Read the model definition and answer for the solid it produces. Units are mm, in the model's axes. A direction names the side the tool comes from. Round coordinates to 2 decimals unless told otherwise and drop trailing zeros. Order: outer loops, then holes, each group sorted by start corner. A loop starts at its lowest first (then second) coordinate and runs counter-clockwise, first axis right, second up. Notation, with made-up numbers: (31, 68.5) -> (49, 68.5) arc R18 ccw to (49, 86.5) -> close; hole circle Ø3 at (39.25, 5). An arc over 180 degrees is marked (long way). One line per item, written item: value. Start each with the question number.
1. Section D-D (x = 122) is taken. Give the vertices of the cut face in (y, z).
2. Consider line 1 (Y direction, x = 39, z = 70.5); line 2 (Z direction, x = -78, y = -39.5); line 3 (X direction, y = -22, z = 64.5). Determine where each line is inside the solid, lowest interval first.
3. Flat-ended cylindrical pins translate along their axes: pin 1 Ø1 at (x, z) = (171.5, 4.5) entering from +Y; pin 2 Ø1 at (x, z) = (-25, 78) entering from +Y; pin 3 Ø1.6 at (y, z) = (-37.5, 128.5) entering from +X; pin 4 Ø6 at (x, z) = (63, 39) entering from -Y. Find the tip coordinate at first contact, or state that the pin passes through.
4. Section C-C (y = -61) is taken. Give the vertices of the cut face in (x, z) (3 decimals).
5. For faces 1 (the face through (-24, -56, 130.175)), 2 (the face through (-8, -38, -3.175)), 3 (the face through (-60.93, -57.73, -1.88)), determine the directions among +Z, -Z, +X, -X, +Y, -Y from which every point of the face is accessible in a straight line to the end or side of a thin tool.
6. Section B-B (z = 38.5) is taken. Give the vertices of the cut face in (x, y), then the cut area to 3 significant figures.
7. Section A-A (x = -29.5) is taken. Give the vertices of the cut face in (y, z) (3 decimals), then the cut area to 3 significant figures.
from build123d import *

# Parameters (mm, degrees)
F5_DEPTH  = 127
F6_W      = 54.5970508829
F6_H      = 20.5464081178
F7_DEPTH  = 3.81
F8_W      = 15.3487510979
F8_H      = 7.4063618667
F8_H_2    = 7.1164776087
F9_DEPTH  = 3.175
F10_W     = 10.7039126975
F10_H     = 8.7776441574
F10_H_2   = 9.3331737444
F11_DEPTH = 3.175
F12_W     = 40.7254230231
F12_H     = 18.2523988187
F12_W_2   = 46.4485138655
F13_DEPTH = 3.175
F14_W     = 15.8928539604
F14_H     = 6.1111226678
F14_W_2   = 13.3333727717
F14_H_2   = 5.5555664003
F15_DEPTH = 3.175
F16_W     = 11.666694656
F16_H     = 5.5555701256
F16_W_2   = 12.222263962
F17_DEPTH = 3.175


# Not quite as in the source:
# - the program builds the solid bodies; features that only make, move or delete a surface that nothing else refers to are left out


with BuildPart() as f5:
    # F0 (on Top) → F5 (new body)
    with BuildSketch(Plane.XY):
        with BuildLine():
            Line((94.2318475405, -7.3630477542), (-68.6407278484, -7.3630477542))
            ThreePointArc((-68.6407278484, -7.3630477542), (-68.7653713247, -7.3626377944), (-68.8900094076, -7.3614079328))
            Line((-68.8900094076, -7.3614079328), (-88.84768188, -7.2301225737))
            Line((-88.84768188, -7.2301225737), (-120.7322572041, -7.2301225737))
            Line((-120.7322572041, -7.2301225737), (-151.5727639198, -17.6438004827))
            Line((-151.5727639198, -17.6438004827), (-151.5727639198, -39.0516258776))
            Line((-151.5727639198, -39.0516258776), (-80.8923020959, -47.3129786551))
            Line((-80.8923020959, -47.3129786551), (-46.3170148432, -70.5671533942))
            Line((-46.3170148432, -70.5671533942), (62.6104325056, -70.5671533942))
            Line((62.6104325056, -70.5671533942), (117.5853461027, -47.3129786551))
            Line((117.5853461027, -47.3129786551), (170.3427284956, -47.3129786551))
            Line((170.3427284956, -47.3129786551), (170.3427284956, -19.2245114595))
            Line((170.3427284956, -19.2245114595), (127.9769688845, -7.2301225737))
            Line((127.9769688845, -7.2301225737), (94.2318475405, -7.3630477542))
        make_face()
    extrude(amount=F5_DEPTH)

    # F6 (on face) → F7 (join)
    with BuildSketch(Plane(origin=(0, 0, 0), x_dir=(1, 0, 0), z_dir=(0, 0, -1))):
        Polygon((-45.8669510931, 67.8593867729), (-76.4162167907, 47.3129786551), (0, 47.3129786551), (0, 67.8593867729), align=None)
        with Locations((35.3119070642, 57.586182714)):
            Rectangle(F6_W, F6_H)
    extrude(amount=F7_DEPTH)

    # F8 (on face) → F9 (join)
    with BuildSketch(Plane.YZ.offset(170.3427284956)):
        with Locations((-39.6386031061, 3.7031809334)):
            Rectangle(F8_W, F8_H)
        with Locations((-39.6386031061, 123.4417611957)):
            Rectangle(F8_W, F8_H_2)
    extrude(amount=F9_DEPTH)

    # F10 (on face) → F11 (join)
    with BuildSketch(Plane(origin=(-151.5727639198, 0, 0), x_dir=(0, -1, 0), z_dir=(-1, 0, 0))):
        with Locations((33.6996695289, 122.6111779213)):
            Rectangle(F10_W, F10_H)
        with Locations((33.6996695289, 4.6665868722)):
            Rectangle(F10_W, F10_H_2)
    extrude(amount=F11_DEPTH)

    # F12 (on face) → F13 (join)
    with BuildSketch(Plane.XY.offset(127)):
        with Locations((42.2477209941, -56.4391780645)):
            Rectangle(F12_W, F12_H)
        with Locations((-23.2242569327, -56.4391780645)):
            Rectangle(F12_W_2, F12_H)
    extrude(amount=F13_DEPTH)

    # F14 (on face) → F15 (join)
    with BuildSketch(Plane(origin=(0, 0, 0), x_dir=(1, 0, 0), z_dir=(0, 0, -1))):
        with Locations((-7.9464269802, 38.065303117)):
            Rectangle(F14_W, F14_H)
        with Locations((56.3295595348, 37.7875249833)):
            Rectangle(F14_W_2, F14_H_2)
    extrude(amount=F15_DEPTH)

    # F16 (on face) → F17 (join)
    with BuildSketch(Plane.XY.offset(127)):
        with Locations((27.7183568105, -38.3430793881)):
            Rectangle(F16_W, F16_H)
        with Locations((-41.4484944195, -38.3430793881)):
            Rectangle(F16_W_2, F16_H)
    extrude(amount=F17_DEPTH)


solid = f5.part
Answer:
1. outline: (-47.31, 0) -> (-7.25, 0) -> (-7.25, 127) -> (-47.31, 127) -> close
2. line 1: -70.57 to -7.36
2. line 2: 0 to 127
2. line 3: -151.57 to 170.34
3. pin 1: y = -31.96
3. pin 2: y = -7.36
3. pin 3: x = 33.55
3. pin 4: y = -70.57
4. outline: (-60.542, 0) -> (-56.066, 0) -> (-56.066, -3.81) -> (0, -3.81) -> (0, 0) -> (8.013, 0) -> (8.013, -3.81) -> (62.61, -3.81) -> (62.61, 0) -> (85.228, 0) -> (85.228, 127) -> (62.61, 127) -> (62.61, 130.175) -> (21.885, 130.175) -> (21.885, 127) -> (0, 127) -> (0, 130.175) -> (-46.449, 130.175) -> (-46.449, 127) -> (-60.542, 127) -> close
5. face 1: +Z, +X, -X, +Y, -Y
5. face 2: -Z, +X, -X, +Y
5. face 3: -Z, -X, -Y
6. outline: (-151.57, -39.05) -> (-80.89, -47.31) -> (-46.32, -70.57) -> (62.61, -70.57) -> (117.59, -47.31) -> (170.34, -47.31) -> (170.34, -19.22) -> (127.98, -7.23) -> (94.23, -7.36) -> (-68.64, -7.36) arc R18.95 cw to (-68.89, -7.36) -> (-88.85, -7.23) -> (-120.73, -7.23) -> (-151.57, -17.64) -> close
6. area: 15,700 mm^2
7. outline: (-70.567, 0) -> (-67.859, 0) -> (-67.859, -3.81) -> (-47.313, -3.81) -> (-47.313, 0) -> (-7.363, 0) -> (-7.363, 127) -> (-47.313, 127) -> (-47.313, 130.175) -> (-65.565, 130.175) -> (-65.565, 127) -> (-70.567, 127) -> close
7. area: 8,160 mm^2
